Build history of the part. All positions in model axes, mm. A direction names the side the tool comes from. Coordinates: 2 decimals unless noted, no trailing zeros. Loops run counter-clockwise (first coordinate to the right, second up) from the corner with the lowest first, then second, coordinate; pieces in that order, holes last.
Item 1: 3-axis set-ups, long thin cutter, end or side, ignore diameter. For faces 5 (the face through (3.461, 6.654, 9.025)), 6 (the face through (0.1, -1.11, 16.01)), 7 (the face through (-1.25, 0, 5)), 8 (the face through (4, 0, 0)), 9 (the face through (-1.25, 0, 23)): which of +Z, -Z, +X, -X, +Y, -Y reach the whole face in a straight line?
Item 2: Cut at B-B (x = 0). List the corners of the cut face in (y, z).
Item 3: Drill centre lines: line 1 along Y through (x, z) = (1.25, 15); line 2 along Z through (x, y) = (3, 0); line 3 along Z through (x, y) = (-8.25, -3.5). Where is each one in solid material? Low to high.
Item 4: Cut at D-D (z = 15). List the corners of the cut face in (x, y).
Item 5: Flat gauge pins, fed straight in: pin 1 (5 mm diameter, centred on y = -6.5, z = 12.5, fed in from -X); pin 2 (3 mm diameter, centred on x = 6.5, z = 14, fed in from -Y); pin 3 (1.3 mm diameter, centred on y = -3, z = 22, fed in from +X); pin 4 (1.8 mm diameter, centred on y = 0, z = 15, fed in from -X). Where does each tip first touch, or does it go through?
Item 6: Mould opens along X. For faces 1 (the face through (-5, 6, 17.8)), 2 (the face through (1.25, 0, 5)), 3 (the face through (-2.124, 9.567, 21.197)), 4 (the face through (1.25, 0, 23)) say: released by +X, released by -X, zero draft, split by the parting line, or undercut.
Item 7: Cut at A-A (y = 0). List the corners of the cut face in (x, z), and give its area (3 significant figures).
Item 8: Cut at C-C (z = 8.5). List the corners of the cut face in (x, y).
from build123d import *

# Parameters (mm, degrees)
F3_DEPTH = 4.2
F4_R     = 0.5
F5_W     = 2.5
F5_H     = 20
F6_DEPTH = 10
F7_R     = 1.5
F8_DEPTH = 12.5


with BuildPart() as f1:
    # F0 (on Front) → F1 (revolve)
    with BuildSketch(Plane.XZ):
        Polygon((0, 25), (0, 0), (7.5, 0), (7.5, 17.8), (9.8, 17.8), (9.8, 25), align=None)
    revolve(axis=Axis((0, 0, 12.5), (0, 0, -1)))

    # F2 (on face) → F3 (cut)
    with BuildSketch(Plane.XY.offset(25)):
        with BuildLine():
            Line((1.25, 15), (-1.25, 15))
            Line((-1.25, 15), (-1.25, 9.7199537036))
            ThreePointArc((-1.25, 9.7199537036), (0, 9.8), (1.25, 9.7199537036))
            Line((1.25, 9.7199537036), (1.25, 15))
        make_face()
        with BuildLine():
            ThreePointArc((1.25, 9.7199537036), (0, 9.8), (-1.25, 9.7199537036))
            Line((-1.25, 9.7199537036), (-1.25, -9.7199537036))
            ThreePointArc((-1.25, -9.7199537036), (0, -9.8), (1.25, -9.7199537036))
            Line((1.25, -9.7199537036), (1.25, 9.7199537036))
        make_face()
        with BuildLine():
            ThreePointArc((1.25, -9.7199537036), (0, -9.8), (-1.25, -9.7199537036))
            Line((-1.25, -9.7199537036), (-1.25, -15))
            Line((-1.25, -15), (1.25, -15))
            Line((1.25, -15), (1.25, -9.7199537036))
        make_face()
    extrude(amount=-F3_DEPTH, mode=Mode.SUBTRACT)

    # F4
    f4_edges = [f1.edges().sort_by_distance(p)[0] for p in [
        (-9.8, 0, 25),
        (7.358329, -6.472635, 25),
        (7.358329, 6.472635, 25),
    ]]
    fillet(f4_edges, radius=F4_R)

    # F5 (on face) → F6 (cut)
    with BuildSketch(Plane(origin=(0, 0, 0), x_dir=(1, 0, 0), z_dir=(0, 0, -1))):
        Rectangle(F5_W, F5_H)
    extrude(amount=-F6_DEPTH, mode=Mode.SUBTRACT)

    # F7 (on Right) → F8 (cut, symmetric)
    with BuildSketch(Plane.YZ):
        with Locations((0, 15)):
            Circle(F7_R)
    extrude(amount=F8_DEPTH, both=True, mode=Mode.SUBTRACT)


solid = f1.part
Filled sheet:
1. face 5: -Z
1. face 6: +X, -X
1. face 7: -Z, +Y, -Y
1. face 8: -Z, +X, -X, +Y, -Y
1. face 9: +Z, +Y, -Y
2. outline: (-9.8, 17.8) - (-7.5, 17.8) - (-7.5, 10) - (7.5, 10) - (7.5, 17.8) - (9.8, 17.8) - (9.8, 20.8) - (-9.8, 20.8) - close; hole circle Ø3 at (0, 15)
3. line 1: y = -7.4 to -1.5, 1.5 to 7.4
3. line 2: z = 0 to 13.5, 16.5 to 25
3. line 3: z = 17.8 to 25
4. outline: (-7.35, -1.5) arc R7.5 ccw to (7.35, -1.5) - close; (-7.35, 1.5) - (7.35, 1.5) arc R7.5 ccw to start
5. pin 1: stops at x = -6.34
5. pin 2: stops at y = -5.59
5. pin 3: stops at x = 9.51
5. pin 4: passes through
6. face 1: zero draft
6. face 2: undercut
6. face 3: split by the parting line
6. face 4: undercut
7. outline: (-9.8, 17.8) - (-7.5, 17.8) - (-7.5, 16.5) - (7.5, 16.5) - (7.5, 17.8) - (9.8, 17.8) - (9.8, 24.5) arc R0.5 ccw to (9.3, 25) - (1.25, 25) - (1.25, 20.8) - (-1.25, 20.8) - (-1.25, 25) - (-9.3, 25) arc R0.5 ccw to (-9.8, 24.5) - close; (-7.5, 0) - (-1.25, 0) - (-1.25, 10) - (1.25, 10) - (1.25, 0) - (7.5, 0) - (7.5, 13.5) - (-7.5, 13.5) - close
7. area: 328 mm2
8. outline: (-1.25, -7.4) - (-1.25, 7.4) arc R7.5 ccw to start; (1.25, -7.4) arc R7.5 ccw to (1.25, 7.4) - close
